Design review of the part shown in the three views and the two pictorial views. Dimensions are in mm from the part's minimum x, y and z. Round coordinates to 2 decimals unless told otherwise and drop trailing zeros. Loops run counter-clockwise (first coordinate to the right, second up) from the corner with the lowest first, then second, coordinate; pieces in that order, holes last. Notation, with made-up numbers: (53, 84) -> (109, 84) arc R16 ccw to (109, 91) -> close; hole circle Ø5 at (4.25, 37.25). An arc over 180 degrees is marked (long way). Return JSON: item names as keys, results as strings. Group by question number.
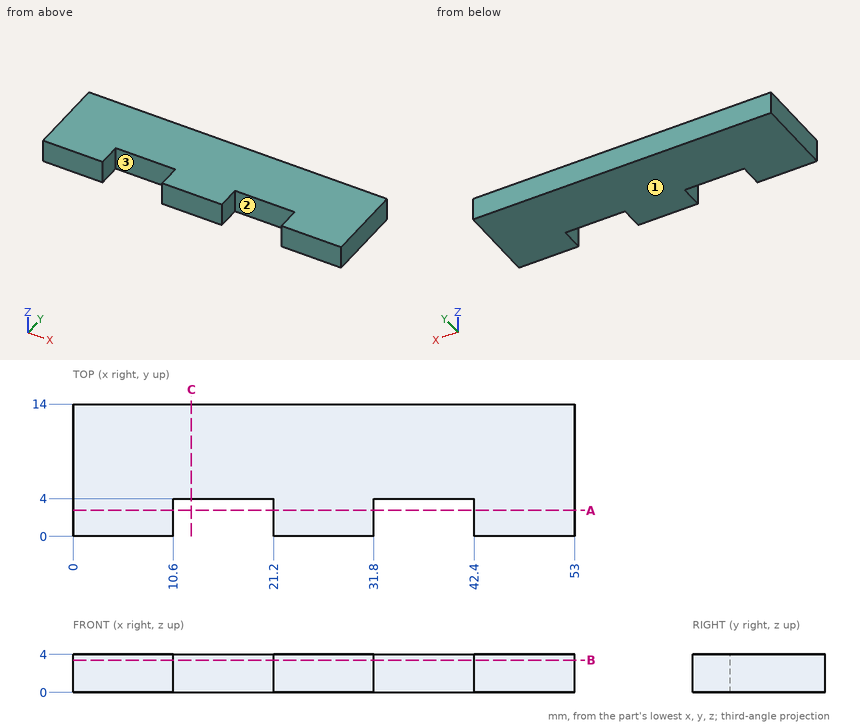
1. We need section A-A, the plane y = 2.75. Write out the cut boundary in (x, z), then the cut area to 3 significant figures.
2. Wall thickness on line 1 (X direction, y = 1.25, z = 3.7); line 2 (Y direction, x = 37, z = 2.6): over which ranges is each line inside the solid? List them lowest first.
3. Draft analysis for pull direction X (two halves, no side actions). For the marked faces 1, 2 and 3, state which applies: pulls with the +X half, pulls with the -X half, needs draft (parallel to the pull), parting line crosses it, or undercut.
4. We need section B-B, the plane z = 3.4. Write out the cut boundary in (x, y).
5. For P1, Ø1.2, axis at x = 38, z = 1, coming from the -Y side, flat-tipped, find the tip position at first contact; note if it passes through.
6. We need section C-C, the plane x = 12.5. Write out the cut boundary in (y, z), then the cut area to 3 significant figures.
Check sheet entries:
{
 "1": {"outline": "(0, 0) -> (10.6, 0) -> (10.6, 4) -> (0, 4) -> close; (21.2, 0) -> (31.8, 0) -> (31.8, 4) -> (21.2, 4) -> close; (42.4, 0) -> (53, 0) -> (53, 4) -> (42.4, 4) -> close", "area": "127 mm²"},
 "2": {"line 1": "x = 0 to 10.6, 21.2 to 31.8, 42.4 to 53", "line 2": "y = 4 to 14"},
 "3": {"face 1": "needs draft", "face 2": "undercut", "face 3": "undercut"},
 "4": {"outline": "(0, 0) -> (10.6, 0) -> (10.6, 4) -> (21.2, 4) -> (21.2, 0) -> (31.8, 0) -> (31.8, 4) -> (42.4, 4) -> (42.4, 0) -> (53, 0) -> (53, 14) -> (0, 14) -> close"},
 "5": {"P1": "stops at y = 4"},
 "6": {"outline": "(4, 0) -> (14, 0) -> (14, 4) -> (4, 4) -> close", "area": "40.0 mm²"}
}
